Design review of the part built by this model. Coordinates are the model's own, in mm. Face numbers are marked on the shaded views. A direction names the side the tool comes from. Give positions to 0.01 mm unless a question says otherwise; leave off trailing zeros. Write each loop counter-clockwise with the first axis right and the second up, starting at its lowest first coordinate (ties: lowest second). Pieces come first, ordered by that corner, then holes.
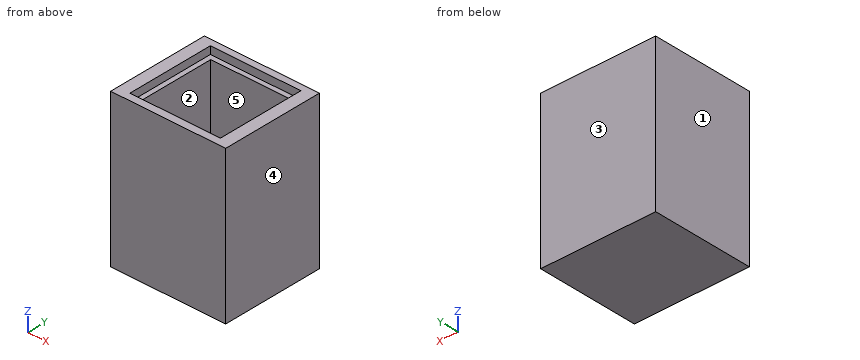
Autodesk Inventor part; units mm, degrees
ref_plane "XZ Plane" through (0, 0, 0) normal (0, 1, 0) x (-1, 0, 0)
ref_plane "XY Plane" through (0, 0, 0) normal (0, 0, 1) x (1, 0, 0)
sketch "Sketch1" plane through (0, 0, 0) normal (0, 0, 1) x (1, 0, 0)
  line L0 (-9.4982, 16.8551) -> (9.4982, 16.8551)
  line L1 (9.4982, 16.8551) -> (9.4982, 0)
  line L2 (9.4982, 0) -> (-9.4982, 0)
  line L3 (-9.4982, 0) -> (-9.4982, 16.8551)
  point P0 (0, 0)
  point P1 (0, 0)
  dimension "d0" = 16.8551
  dimension "d1" = 18.9965
extrude "Extrusion1" add sketch "Sketch1" along normal mid plane 25.4
sketch "Sketch2" plane through (0, 0, 12.7) normal (0, 0, 1) x (1, 0, 0)
  line L0 (-6.666, 14.9209) -> (6.666, 14.9209)
  line L1 (6.666, 14.9209) -> (6.666, 2.0723)
  line L2 (6.666, 2.0723) -> (-6.666, 2.0723)
  line L3 (-6.666, 2.0723) -> (-6.666, 14.9209)
  line L4 (-9.4982, 0) -> (9.4982, 0)
  point P0 (0, 0)
  point P1 (0, 0)
  point P2 (0, 2.0723)
  dimension "d4" = 12.8485
  dimension "d5" = 13.3321
extrude "Extrusion2" cut sketch "Sketch2" against normal blind 22.86
ref_plane "Work Plane1" through (0, 0, 0) normal (1, 0, 0) x (0, 1, 0)
sketch "Sketch3" plane through (0, 0, 0) normal (1, 0, 0) x (0, 1, 0)
  line L0 (14.9209, 12.7) -> (14.9209, -10.16)
  line L1 (16.8551, 12.7) -> (0, 12.7)
  line L2 (15.7291, 12.7) -> (15.7291, 11.4381)
  line L3 (15.7291, 11.4381) -> (14.9209, 11.4381)
  line L4 (14.9209, 11.4381) -> (14.9209, 12.7)
  line L5 (15.7291, 12.7) -> (14.9209, 12.7)
  point P0 (0, 0)
  dimension "d9" = 1.2619
  dimension "d10" = 0.8082
sketch3d "3D Sketch1"
  line L0 (-6.666, 14.9209, 12.7) -> (-6.666, 2.0723, 12.7)
  line L1 (-6.666, 2.0723, 12.7) -> (6.666, 2.0723, 12.7)
  line L2 (6.666, 2.0723, 12.7) -> (6.666, 14.9209, 12.7)
  line L3 (6.666, 14.9209, 12.7) -> (-6.666, 14.9209, 12.7)
sweep "Sweep1" cut profiles "Sketch3" path "3D Sketch1"
(1) Consider section A-A, the plane x = -1.5. Give the boundary of the cut face in (y, z).
Resolved:
outline: (0, -12.7) - (16.86, -12.7) - (16.86, 12.7) - (15.73, 12.7) - (15.73, 11.44) - (14.92, 11.44) - (14.92, -10.16) - (2.07, -10.16) - (2.07, 11.44) - (1.26, 11.44) - (1.26, 12.7) - (0, 12.7) - close
(2) Tool access review of the marked faces 4 and 5: name each direction out of +Z, -Z, +X, -X, +Y, -Y from which nothing blocks a thin tool from reaching the whole face with its end or side.
Resolved:
face 4: +Z, -Z, +X, +Y, -Y
face 5: +Z
(3) To check wall thickness, follow L1, parallel to Y at x = 3, z = 1.5; L2, parallel to X at y = 6.75, z = -4.5; L3, parallel to Z at x = 2.5, y = 3.75. State the ranges of each line that lie inside material, in increasing order.
Resolved:
L1: y = 0 to 2.07, 14.92 to 16.86
L2: x = -9.5 to -6.67, 6.67 to 9.5
L3: z = -12.7 to -10.16
(4) Consider section B-B, the plane y = 8.75. Give the boundary of the cut face in (x, z).
Resolved:
outline: (-9.5, -12.7) - (9.5, -12.7) - (9.5, 12.7) - (7.47, 12.7) - (7.47, 11.44) - (6.67, 11.44) - (6.67, -10.16) - (-6.67, -10.16) - (-6.67, 11.44) - (-7.47, 11.44) - (-7.47, 12.7) - (-9.5, 12.7) - close
(5) Mouldability with a two-part tool opening along Y and no side actions: class the marked faces 1, 2 and 3 as pulls with the +Y half, pulls with the -Y half, needs draft (parallel to the pull), parting line crosses it, or undercut.
Resolved:
face 1: needs draft
face 2: undercut
face 3: pulls with the +Y half
(6) Consider section D-D, the plane x = -7. Give the boundary of the cut face in (y, z).
Resolved:
outline: (0, -12.7) - (16.86, -12.7) - (16.86, 12.7) - (15.73, 12.7) - (15.73, 11.44) - (1.26, 11.44) - (1.26, 12.7) - (0, 12.7) - close
(7) Consider section C-C, the plane z = -0.5. Give the boundary of the cut face in (x, y).
Resolved:
outline: (-9.5, 0) - (9.5, 0) - (9.5, 16.86) - (-9.5, 16.86) - close; hole (-6.67, 2.07) - (6.67, 2.07) - (6.67, 14.92) - (-6.67, 14.92) - close
